from build123d import *

# Parameters (mm, degrees)
SKETCH1_R           = 20.32
OUTER_CIRCLE_DEPTH  = 6.35
TOOTH_CUT_DEPTH     = 30.430040775
TEETH_PATTERN_COUNT = 30
CUT_EXTRUDE1_DEPTH  = 30.382561533


with BuildPart() as part:
    # Sketch1 → Outer Circle (new body)
    with BuildSketch(Plane.XY):
        Circle(SKETCH1_R)
    extrude(amount=OUTER_CIRCLE_DEPTH)

    # Sketch2 → Tooth Cut (cut, through all)
    with BuildSketch(Plane.XY.offset(6.35)):
        with BuildLine():
            ThreePointArc((-0.743845606, 17.764433391), (0, 17.78), (0.743845606, 17.764433391))
            ThreePointArc((0.743845606, 17.764433391), (1.009950749, 19.081439594), (1.671040922, 20.251173355))
            ThreePointArc((1.671040922, 20.251173355), (0, 20.32), (-1.671040922, 20.251173355))
            ThreePointArc((-1.671040922, 20.251173355), (-1.009950749, 19.081439594), (-0.743845606, 17.764433391))
        make_face()
    tooth_cut = extrude(amount=-TOOTH_CUT_DEPTH, mode=Mode.SUBTRACT)

    # Teeth Pattern: Tooth Cut ×30 about axis
    teeth_pattern_axis = Axis((0, 0, 0), (0, 0, 1))
    for i in range(1, TEETH_PATTERN_COUNT):
        add(tooth_cut.rotate(teeth_pattern_axis, i * 360 / TEETH_PATTERN_COUNT), mode=Mode.SUBTRACT)

    # Sketch3 → Cut-Extrude1 (cut, through all)
    with BuildSketch(Plane.XY.offset(6.35)):
        with BuildLine():
            Line((0, 2.31775), (-2.141974636, 2.31775))
            ThreePointArc((-2.141974636, 2.31775), (-2.938938883, -1.150068974), (0, -3.15595))
            Line((0, -3.15595), (0, 2.31775))
        make_face()
        with BuildLine():
            Line((2.141974636, 2.31775), (0, 2.31775))
            Line((0, 2.31775), (0, -3.15595))
            ThreePointArc((0, -3.15595), (2.231593646, -2.231593646), (3.15595, 0))
            ThreePointArc((3.15595, 0), (2.891365184, 1.264922043), (2.141974636, 2.31775))
        make_face()
    extrude(amount=-CUT_EXTRUDE1_DEPTH, mode=Mode.SUBTRACT)


solid = part.part
Geometry: final body of the model. Coordinates: model frame, mm. A direction names the side the tool comes from. Round coordinates to 2 decimals unless told otherwise and drop trailing zeros. Order: outer loops, then holes, each group sorted by start corner. A loop starts at its lowest first (then second) coordinate and runs counter-clockwise, first axis right, second up.
Q1. Pin query (flat end, axial travel): pin 1 (2 mm diameter, centred on x = 9.5, z = 3, fed in from -Y). Return the tip coordinate at first contact, or that it passes through.
Result sheet:
pin 1: stops at y = -17.82
Q2. Section A-A, the plane x = -9. Output: boundary loops of the cut face in (y, z), and give its area (3 significant figures).
Result sheet:
outline: (-17.31, 0) - (17.31, 0) - (17.31, 6.35) - (-17.31, 6.35) - close
area: 220 mm2
Q3. Material intervals for probe 1 along Y at (x, z) = (10, 3); probe 2 along Y at (x, z) = (19.5, 1.5); probe 3 along Y at (x, z) = (18, 1), sorted ascending.
Result sheet:
probe 1: y = -17.69 to -15.07, -14.7 to 14.7, 15.07 to 17.69
probe 2: y = -4.76 to -3.38, -0.86 to 0.86, 3.38 to 4.76
probe 3: y = -8.72 to -6.99, -4.93 to -2.68, -1.13 to 1.13, 2.68 to 4.93, 6.99 to 8.72
Q4. Access query for faces 1 (the face through (-8.697, 17.034, 3.219)), 2 (the face through (0, 2.318, 3)), 3 (the face through (-16.008, 10.401, 3.219)), 4 (the face through (-4.945, -18.439, 3.219)). Directions: +Z, -Z, +X, -X, +Y, -Y. A direction counts if a zero-diameter tool reaches every point of the face in a straight line with its end or side. Return the directions, or none.
Result sheet:
face 1: +Z, -Z, +Y
face 2: +Z, -Z
face 3: +Z, -Z, -X
face 4: +Z, -Z, -Y
Q5. Mould query, pull axis X, two halves, no side actions, for faces 5 (the face through (-17.821, 6.845, 3.219)), 6 (the face through (0, -4, 0)), 7 (the face through (-2.977, -18.893, 3.219)), 8 (the face through (7.22, 16.25, 3.22)). Classes: released by +X, released by -X, zero draft, split by the parting line, or undercut.
Result sheet:
face 5: released by -X
face 6: zero draft
face 7: undercut
face 8: undercut
